The model under review builds one solid part; all positions refer to its coordinate system, in mm. A direction names the side the tool comes from. Round coordinates to 2 decimals unless told otherwise and drop trailing zeros. Loops run counter-clockwise (first coordinate to the right, second up) from the corner with the lowest first, then second, coordinate; pieces in that order, holes last. Notation, with made-up numbers: M 18,77.25 L 54,77.25 A30 cw 54,112.25 Z; hole C 30,-3.5 d7. An arc over 180 degrees is marked long. Answer as a JSON object with one key per item and string values. Group by question number.
Item 1: Tool access review of faces 1 (the face through (11.07, -25.67, 80.54)), 2 (the face through (-7, -12, 17)), 3 (the face through (0, -6, -6)), 4 (the face through (6, -8, 65)): name each direction out of +Z, -Z, +X, -X, +Y, -Y from which nothing blocks a thin tool from reaching the whole face with its end or side.
Item 2: Consider section D-D (z = 67). Give the boundary of the cut face in (x, y), and give its area (3 significant figures).
Item 3: The part is to be moulded in two halves that separate along Z. For faces 5 (the face through (0, -6, 45)), 6 (the face through (11.07, -15.78, 75.95)), 7 (the face through (-10.93, -25.67, 80.54)), say which applies: +Z half, -Z half, draft (parallel to the pull), parting line (faces both ways), or undercut.
Item 4: Consider section C-C (z = 30). Give the boundary of the cut face in (x, y).
Item 5: Consider section B-B (y = -18). Give the boundary of the cut face in (x, z), and give its area (3 significant figures).
Item 6: Insertion check: P1, Ø10, axis at x = -5, z = 6, coming from the -Y side; P2, Ø9.5, axis at y = -15, z = 70, coming from the -X side; P3, Ø5, axis at x = 6, y = -19.5, coming from the +Z side; P4, Ø14, axis at y = -15, z = 70, coming from the +X side. Each pin has a flat end and moves straight along its axis. Give the tip position at first contact, or say it passes through.
Item 7: To check wall thickness, follow line 1 (X direction, y = -6.25, z = 11); line 2 (Z direction, x = 11.5, y = -20.25); line 3 (Z direction, x = 10.25, y = -15). State the ranges of each line that lie inside material, in increasing order.
Item 8: Consider section A-A (x = 0). Give the boundary of the cut face in (y, z).
```python
from build123d import *

# Parameters (mm, degrees)
F1_DEPTH = 30
F3_DEPTH = 50
F2_R     = 6
F4_DEPTH = 25.5


# Not quite as in the source:
# - a feature of the source that left no trace in its solid (it failed there, or was rolled back) is left out


with BuildPart() as f1:
    # F0 (on Front) → F1 (new body)
    with BuildSketch(Plane.XZ):
        with BuildLine():
            Line((-16, 85), (-16, 0))
            ThreePointArc((-16, 0), (0, -16), (16, 0))
            Line((16, 0), (16, 85))
            Line((16, 85), (6, 85))
            Line((6, 85), (6, 45))
            Line((6, 45), (-6, 45))
            Line((-6, 45), (-6, 85))
            Line((-6, 85), (-16, 85))
        make_face()
        with BuildLine():
            ThreePointArc((6, 1.3e-09), (-0.0001359155, -5.9999999985), (-5.9999999938, 0.0002718323))
            Line((-5.9999999938, 0.0002718323), (-5.9988673594, 25.0002718323))
            ThreePointArc((-5.9988673594, 25.0002718323), (0.0014044667, 30.9999999938), (6.0011326283, 24.9997281677))
            Line((6.0011326283, 24.9997281677), (6.0000000062, 0))
        make_face(mode=Mode.SUBTRACT)
    extrude(amount=F1_DEPTH)

    # F2 (on Right) → F3 (cut, symmetric)
    with BuildSketch(Plane.YZ):
        with BuildLine():
            ThreePointArc((-15.7894736842, 55.0207900308), (-25.8821437517, 59.6762919758), (-30, 70))
            Line((-30, 70), (-30, -16))
            Line((-30, -16), (-12, -16))
            Line((-12, -16), (-12, 51.026334039))
            ThreePointArc((-12, 51.026334039), (-13.0980949996, 53.7793228454), (-15.7894736842, 55.0207900308))
        make_face()
        with BuildLine():
            Line((-30, 85), (-30, 70))
            ThreePointArc((-30, 70), (-25.6066016991, 80.6066017365), (-14.9999999471, 85))
            Line((-14.9999999471, 85), (-30, 85))
        make_face()
        with BuildLine():
            Line((0, 85), (-14.9999999471, 85))
            ThreePointArc((-14.9999999471, 85), (-4.3933982635, 80.6066016991), (0, 70))
            Line((0, 70), (0, 85))
        make_face()
    extrude(amount=F3_DEPTH, both=True, mode=Mode.SUBTRACT)

    # F2 (on Right) → F4 (cut, symmetric)
    with BuildSketch(Plane.YZ):
        with Locations((-15, 70)):
            Circle(F2_R)
    extrude(amount=F4_DEPTH, both=True, mode=Mode.SUBTRACT)


solid = f1.part
```
Geometry results:
{
 "1": {"face 1": "+X, -X", "face 2": "-Z, +X, -X, -Y", "face 3": "+Y, -Y", "face 4": "+Z, +Y, -Y"},
 "2": {"outline": "M -16,-29.7 L -6,-29.7 L -6,-20.2 L -16,-20.2 Z; M -16,-9.8 L -6,-9.8 L -6,0 L -16,0 Z; M 6,-29.7 L 16,-29.7 L 16,-20.2 L 6,-20.2 Z; M 6,-9.8 L 16,-9.8 L 16,0 L 6,0 Z", "area": "386 mm^2"},
 "3": {"face 5": "+Z half", "face 6": "undercut", "face 7": "parting line"},
 "4": {"outline": "M -16,-12 L -3.32,-12 L -3.32,0 L -16,0 Z; M 3.32,-12 L 16,-12 L 16,0 L 3.32,0 Z"},
 "5": {"outline": "M -16,55.3 L -6,55.3 L -6,64.8 L -16,64.8 Z; M -16,75.2 L -6,75.2 L -6,84.7 L -16,84.7 Z; M 6,55.3 L 16,55.3 L 16,64.8 L 6,64.8 Z; M 6,75.2 L 16,75.2 L 16,84.7 L 6,84.7 Z", "area": "380 mm^2"},
 "6": {"P1": "stops at y = -12", "P2": "passes through", "P3": "stops at z = 84.87", "P4": "stops at x = 16"},
 "7": {"line 1": "x = -16 to -6, 6 to 16", "line 2": "z = 55.95 to 67.1, 72.9 to 84.05", "line 3": "z = 54.9 to 64, 76 to 85"},
 "8": {"outline": "M -12,-16 L 0,-16 L 0,-6 L -12,-6 Z; M -12,31 L 0,31 L 0,45 L -12,45 Z"}
}
